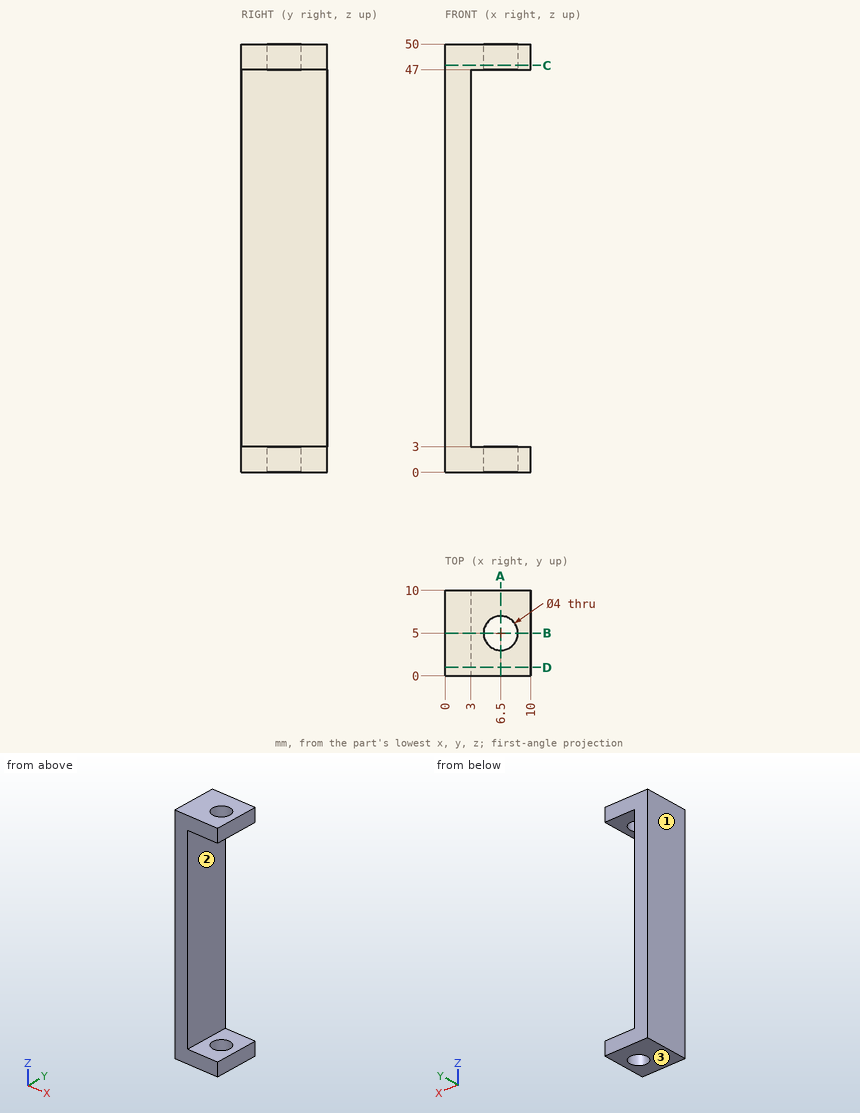
The drawing under review shows one solid part. Ordinate dimensions are in mm from its lowest x, y, z. Round coordinates to 2 decimals unless told otherwise and drop trailing zeros. Order: outer loops, then holes, each group sorted by start corner. A loop starts at its lowest first (then second) coordinate and runs counter-clockwise, first axis right, second up. Notation, with made-up numbers: (59, 83.25) - (95, 83.25) arc R22 ccw to (95, 99.25) - close; hole circle Ø11 at (85, 40). An arc over 180 degrees is marked (long way). Return JSON: item names as keys, results as strings.
Q1. For pin 1 Ø6 at (x, z) = (4, 22) entering from -Y; pin 2 Ø2 at (x, z) = (5.5, 26) entering from +Y; pin 3 Ø6 at (y, z) = (5, 9) entering from +X, all flat-tipped, find the tip position at first contact; note any pin that passes through.
Computed values:
{"pin 1": "stops at y = 0", "pin 2": "passes through", "pin 3": "stops at x = 3"}
Q2. The part is to be moulded in two halves that separate along Z. For the marked faces 1, 2 and 3, say which applies: pulls with the +Z half, pulls with the -Z half, needs draft (parallel to the pull), parting line crosses it, or undercut.
Computed values:
{"face 1": "needs draft", "face 2": "undercut", "face 3": "pulls with the -Z half"}
Q3. Consider section B-B on y = 5. Write out the cut boundary in (x, z).
Computed values:
{"outline": "(0, 0) - (4.5, 0) - (4.5, 3) - (3, 3) - (3, 47) - (4.5, 47) - (4.5, 50) - (0, 50) - close; (8.5, 0) - (10, 0) - (10, 3) - (8.5, 3) - close; (8.5, 47) - (10, 47) - (10, 50) - (8.5, 50) - close"}
Q4. Consider section A-A on x = 6.5. Write out the cut boundary in (y, z), plus the area to 3 significant figures.
Computed values:
{"outline": "(0, 0) - (3, 0) - (3, 3) - (0, 3) - close; (0, 47) - (3, 47) - (3, 50) - (0, 50) - close; (7, 0) - (10, 0) - (10, 3) - (7, 3) - close; (7, 47) - (10, 47) - (10, 50) - (7, 50) - close", "area": "36.0 mm2"}
Q5. Consider section C-C on z = 47.5. Write out the cut boundary in (x, y), plus the area to 3 significant figures.
Computed values:
{"outline": "(0, 0) - (10, 0) - (10, 10) - (0, 10) - close; hole circle Ø4 at (6.5, 5)", "area": "87.4 mm2"}
Q6. Wall thickness on L1, parallel to Z at x = 7.75, y = 8.25; L2, parallel to Y at x = 6.5, z = 49.45; L3, parallel to X at y = 8.25, z = 19: over which ranges is each line inside the solid? List them lowest first. Write a range as [from, to].
Computed values:
{"L1": "z = [0, 3], [47, 50]", "L2": "y = [0, 3], [7, 10]", "L3": "x = [0, 3]"}
Q7. Consider section D-D on y = 1. Write out the cut boundary in (x, z).
Computed values:
{"outline": "(0, 0) - (10, 0) - (10, 3) - (3, 3) - (3, 47) - (10, 47) - (10, 50) - (0, 50) - close"}
